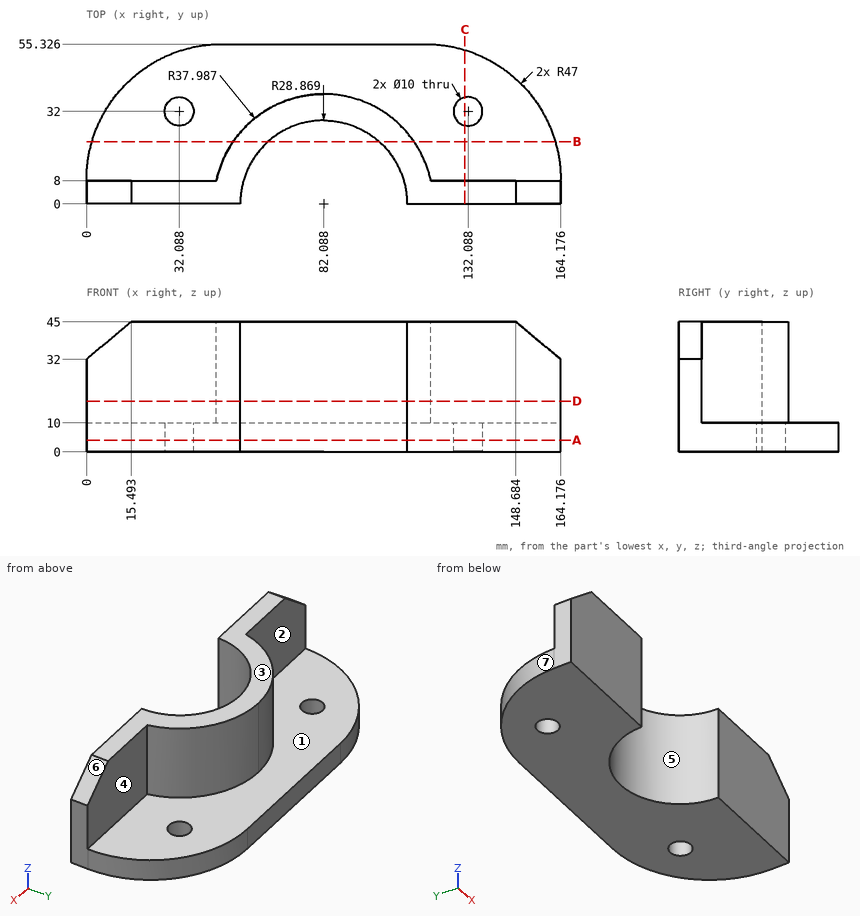
The figure shows three views and two pictorial views of one solid part (mm, origin at its lowest corner). Answer the questions. A direction names the side the tool comes from. Give positions to 0.01 mm unless a question says otherwise; leave off trailing zeros. Loops run counter-clockwise (first coordinate to the right, second up) from the corner with the lowest first, then second, coordinate; pieces in that order, holes last. Notation, with made-up numbers: (61, -39.75) -> (110, -39.75) arc R34 cw to (110, -5.75) -> close; hole circle Ø10 at (-24, -32.75). An arc over 180 degrees is marked (long way). Put each result on its own line as item: value. Start each with the question number.
Item 1: The mould has two halves that part along X. Classify the marked faces 4, 5, 6 and 7: released by +X, released by -X, zero draft, split by the parting line, or undercut.
Item 2: Find the intervals of material crossed by L1, parallel to Y at x = 41.5, z = 35.5; L2, parallel to Z at x = 65.5, y = 42; L3, parallel to Y at x = 118, z = 4.5, in increasing order. Write a range as [from, to].
Item 3: Which of the six approach directions +Z, -Z, +X, -X, +Y, -Y give full straight-line access (tool end or side, diameter ignored) to the marked faces 1, 2 and 3?
Item 4: The part is cut by section A-A (z = 4). Give the vertices of the cut face in (x, y).
Item 5: Each of these flat-tipped pins is pushed along its axis until it touches: P1, Ø3, axis at x = 113.5, z = 17, coming from the +Y side (1 decimal); P2, Ø2, axis at x = 123, z = 10.5, coming from the +Y side; P3, Ø1, axis at x = 44.5, y = 17.5, coming from the +Z side. Where does it stop, or does it pass through?
Item 6: The part is cut by section C-C (x = 131). Give the vertices of the cut face in (y, z).
Item 7: The part is cut by section D-D (z = 17.5). Give the vertices of the cut face in (x, y), then the cut area to 3 significant figures.
Item 8: The part is cut by section B-B (y = 21.5). Give the vertices of the cut face in (x, z) (1 decimal).
Answers below:
1. face 4: zero draft
1. face 5: undercut
1. face 6: released by +X
1. face 7: released by -X
2. L1: [0, 8]
2. L2: [0, 10]
2. L3: [0, 55.32]
3. face 1: +Z, +Y
3. face 2: +Z, -X, +Y
3. face 3: +Z, +X, -X, +Y, -Y
4. outline: (0, 0) -> (53.22, 0) arc R28.87 cw to (110.96, 0) -> (164.18, 0) -> (164.18, 8.33) arc R47 ccw to (117.18, 55.33) -> (47, 55.33) arc R47 ccw to (0, 8.33) -> close; hole circle Ø10 at (32.09, 32); hole circle Ø10 at (132.09, 32)
5. P1: y = 23.4
5. P2: y = 55.06
5. P3: z = 10
6. outline: (0, 0) -> (27.12, 0) -> (27.12, 10) -> (8, 10) -> (8, 45) -> (0, 45) -> close; (36.88, 0) -> (53.25, 0) -> (53.25, 10) -> (36.88, 10) -> close
7. outline: (0, 0) -> (53.22, 0) arc R28.87 cw to (110.96, 0) -> (164.18, 0) -> (164.18, 8) -> (119.22, 8) arc R37.99 ccw to (44.95, 8) -> (0, 8) -> close
7. area: 1,670 mm2
8. outline: (1.9, 0) -> (62.8, 0) -> (62.8, 45) -> (50.8, 45) -> (50.8, 10) -> (1.9, 10) -> close; (101.4, 0) -> (162.3, 0) -> (162.3, 10) -> (113.4, 10) -> (113.4, 45) -> (101.4, 45) -> close
